Verification items for the finished model (mm, model axes). Face numbers are marked on the shaded views. Coordinates: 2 decimals unless noted, no trailing zeros. Order: outer loops, then holes, each group sorted by start corner. A loop starts at its lowest first (then second) coordinate and runs counter-clockwise, first axis right, second up. Notation, with made-up numbers: M 20,51.25 L 37,51.25 A11 ccw 37,57.25 Z; hole C -11,27 d4. An arc over 180 degrees is marked long. Return JSON: item names as keys, results as strings.
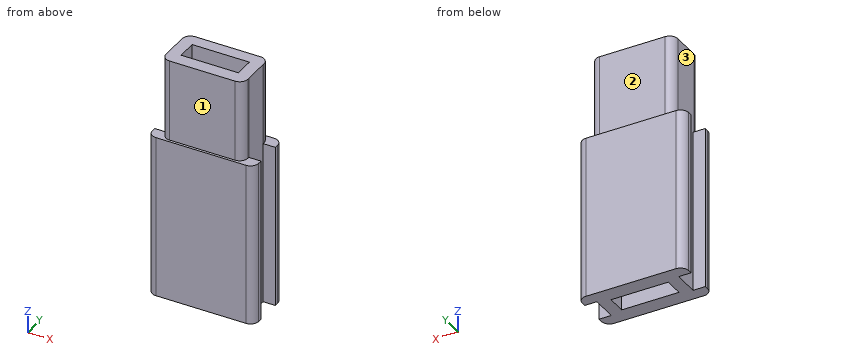
```python
from build123d import *

# Parameters (mm, degrees)
F0_W     = 7
F0_H     = 2.3
F1_DEPTH = 20
F3_DEPTH = 10
F4_R     = 1
F5_R     = 1


with BuildPart() as f1:
    # F0 (on Top) → F1 (new body)
    with BuildSketch(Plane.XY):
        Polygon((6.5, 3.05), (-6.5, 3.05), (-6.5, 1.55), (-5, 1.55), (-5, -1.55), (-6.5, -1.55), (-6.5, -3.05), (6.5, -3.05), (6.5, -1.55), (5, -1.55), (5, 1.55), (6.5, 1.55), align=None)
        Rectangle(F0_W, F0_H, mode=Mode.SUBTRACT)
    extrude(amount=F1_DEPTH)

    # F2 (on face) → F3 (join)
    with BuildSketch(Plane.XY.offset(20)):
        Polygon((-5, -1.55), (-5, -2.75), (5.006821, -2.75), (5.006821, -1.55), (5, -1.55), (5, 1.55), (5.006821, 1.55), (5.006821, 2.75), (-5, 2.75), (-5, 1.55), align=None)
        Polygon((3.5, -1.15), (-3.5, -1.15), (-3.5, 1.15), (-3.5, 1.25), (3.5, 1.25), (3.5, 1.15), align=None, mode=Mode.SUBTRACT)
    extrude(amount=F3_DEPTH)

    # F4
    f4_edges = [f1.edges().sort_by_distance(p)[0] for p in [
        (-5, 2.75, 25),
        (-5, -2.75, 25),
        (5.006821, 2.75, 25),
        (5.006821, -2.75, 25),
    ]]
    fillet(f4_edges, radius=F4_R)

    # F5
    f5_edges = [f1.edges().sort_by_distance(p)[0] for p in [
        (-6.5, 3.05, 10),
        (-6.5, -3.05, 10),
        (6.5, 3.05, 10),
        (6.5, -3.05, 10),
    ]]
    fillet(f5_edges, radius=F5_R)


solid = f1.part
```
Q1. Go/stop test with flat-tipped pins: pin 1 (1.2 mm diameter, centred on y = -0.5, z = 14, fed in from +X); pin 2 (4 mm diameter, centred on x = 0, z = 26, fed in from +Y); pin 3 (3.5 mm diameter, centred on x = 1.5, z = 24, fed in from -Y); pin 4 (3.5 mm diameter, centred on x = 0.5, z = 20.5, fed in from +Y). Record where each tip stops, or that it passes through.
Values:
{"pin 1": "x = 5", "pin 2": "y = 2.75", "pin 3": "y = -2.75", "pin 4": "y = 3.05"}
Q2. Cross-section at B-B, the plane z = 9. Record the boundary of the cut face in (x, y).
Values:
{"outline": "M -6.5,-2.05 A1 ccw -5.5,-3.05 L 5.5,-3.05 A1 ccw 6.5,-2.05 L 6.5,-1.55 L 5,-1.55 L 5,1.55 L 6.5,1.55 L 6.5,2.05 A1 ccw 5.5,3.05 L -5.5,3.05 A1 ccw -6.5,2.05 L -6.5,1.55 L -5,1.55 L -5,-1.55 L -6.5,-1.55 Z; hole M -3.5,-1.15 L 3.5,-1.15 L 3.5,1.15 L -3.5,1.15 Z"}
Q3. Cross-section at C-C, the plane y = 0.75. Record the boundary of the cut face in (x, z), and give its area (3 significant figures).
Values:
{"outline": "M -5,0 L -3.5,0 L -3.5,30 L -5,30 Z; M 3.5,0 L 5,0 L 5,30 L 3.5,30 Z", "area": "90.0 mm^2"}
Q4. Draft check along Y on the marked faces 1, 2 and 3. Enter one of: pulls with the +Y half, pulls with the -Y half, needs draft (parallel to the pull), parting line crosses it, or undercut.
Values:
{"face 1": "pulls with the -Y half", "face 2": "pulls with the +Y half", "face 3": "undercut"}
Q5. Material ranges on line 1 along X through (y, z) = (1, 6.5); line 2 along Y through (x, z) = (-0.75, 16.5); line 3 along Y through (x, z) = (5.25, 17.5), recorded low to high.
Values:
{"line 1": "-5 to -3.5, 3.5 to 5", "line 2": "-3.05 to -1.15, 1.15 to 3.05", "line 3": "-3.05 to -1.55, 1.55 to 3.05"}
Q6. Cross-section at A-A, the plane x = 0.5. Record the boundary of the cut face in (y, z).
Values:
{"outline": "M -3.05,0 L -1.15,0 L -1.15,30 L -2.75,30 L -2.75,20 L -3.05,20 Z; M 1.15,0 L 3.05,0 L 3.05,20 L 2.75,20 L 2.75,30 L 1.25,30 L 1.25,20 L 1.15,20 Z"}
